Could you check a few things on this model? Use its own coordinates, in mm. A direction names the side the tool comes from. Give positions to 0.01 mm unless a question says otherwise; leave off trailing zeros. Use a Markdown table: item, result. Add a question column.
Item 1: I'm going to push flat-ended pins straight in: pin 1 Ø1.5 at (x, y) = (8, 3.5) entering from +Z; pin 2 Ø0.7 at (x, z) = (12.5, -1) entering from +Y. Where does each tip first touch, or does it pass through?
Item 2: For faces 1 (the face through (0, 1, -2)), 2 (the face through (4, 4.59, -1.68)), which set-ups out of +Z, -Z, +X, -X, +Y, -Y let a thin tool reach every point of the face, with its end or its side?
Item 3: If we mould it in two halves opening along X, with no side actions, what happens to faces 3 (the face through (0.86, 4.59, -1.68)), 4 (the face through (43.134, 4.559, -1.676)), 5 (the face through (27, 0, -2))? For each: released by +X, released by -X, zero draft, split by the parting line, or undercut.
Item 4: If I drill on L1, parallel to Y at x = 37.5, z = -2; L2, parallel to X at y = 3.15, z = -2.2, over which ranges is the centre line in solid material (lowest first)? Write a range as from..to.
from build123d import *

# Parameters (mm, degrees)
BLANKSKE_W        = 54.3
BLANKSKE_H        = 5.7
BLANK_DEPTH       = 3.4
TOOTHCUTSIM_DEPTH = 55.704113191
TEETHCUTS_COUNT   = 18
TEETHCUTS_PITCH   = 3.14159265
VERRUNDUNG1_R     = 0.5
VERRUNDUNG2_R     = 0.5


with BuildPart() as part:
    # BlankSke → Blank (new body)
    with BuildSketch(Plane.XY):
        with Locations((27.15, 2.85)):
            Rectangle(BLANKSKE_W, BLANKSKE_H)
    extrude(amount=-BLANK_DEPTH)

    # TooCutSkeSim → ToothCutSim (cut, through all)
    with BuildSketch(Plane.XY):
        Polygon((0.44443537, 3.45), (-0.44443537, 3.45), (-1.272613241, 5.7254), (1.272613241, 5.7254), align=None)
    toothcutsim = extrude(amount=-TOOTHCUTSIM_DEPTH, mode=Mode.SUBTRACT)

    # TeethCuts: ToothCutSim ×18
    with Locations(*[(i * TEETHCUTS_PITCH, 0, 0) for i in range(1, TEETHCUTS_COUNT)]):
        add(toothcutsim, mode=Mode.SUBTRACT)

    # Verrundung1
    # the kernel refuses this fillet: 0.5 mm, written as the material it takes off along each edge
    with BuildSketch(Plane(origin=(54.3, 4.682214995, -7.723886484), x_dir=(0, -1, 0), z_dir=(0, 0, 1))) as verrundung1_piece_1:
        with BuildLine():
            CenterArc((1.729554594, -0.5), VERRUNDUNG1_R, 90, 84.086849411)
            Line((1.232214995, -0.44848958), (1.222268203, -0.447459372))
            ThreePointArc((1.222268203, -0.447459372), (0.612687296, -0.233641716), (-0.003420201, -0.009396926))
            Line((-0.003420201, -0.009396926), (0, 0.01))
            Line((0, 0.01), (1.729554594, 0.01))
            Line((1.729554594, 0.01), (1.729554594, 0))
        make_face()
    extrude(amount=12.047772969, mode=Mode.SUBTRACT)

    # Verrundung2
    # the kernel refuses this fillet: 0.5 mm, written as the material it takes off along each edge
    with BuildSketch(Plane(origin=(0, 3.45, 1.242257451), x_dir=(0, -1, 0), z_dir=(0, 0, -1))) as verrundung2_piece_1:
        with BuildLine():
            CenterArc((0.49690298, -0.5), VERRUNDUNG2_R, 90, 83.619583418)
            Line((0, -0.44443537), (-0.00993806, -0.443324077))
            ThreePointArc((-0.00993806, -0.443324077), (-0.01, -0.222217685), (-0.01, 0))
            Line((-0.01, 0), (0, 0.01))
            Line((0, 0.01), (0.49690298, 0.01))
            Line((0.49690298, 0.01), (0.49690298, 0))
        make_face()
    extrude(amount=5.884514902, mode=Mode.SUBTRACT)


solid = part.part
Findings below:
| question | item | result |
|---|---|---|
| 1 | pin 1 | stops at z = 0 |
| 1 | pin 2 | stops at y = 3.45 |
| 2 | face 1 | +Z, -Z, -X, +Y, -Y |
| 2 | face 2 | +Z, -Z, +Y |
| 3 | face 3 | released by -X |
| 3 | face 4 | undercut |
| 3 | face 5 | zero draft |
| 4 | L1 | y = 0..3.45 |
| 4 | L2 | x = 0.04..54.26 |
